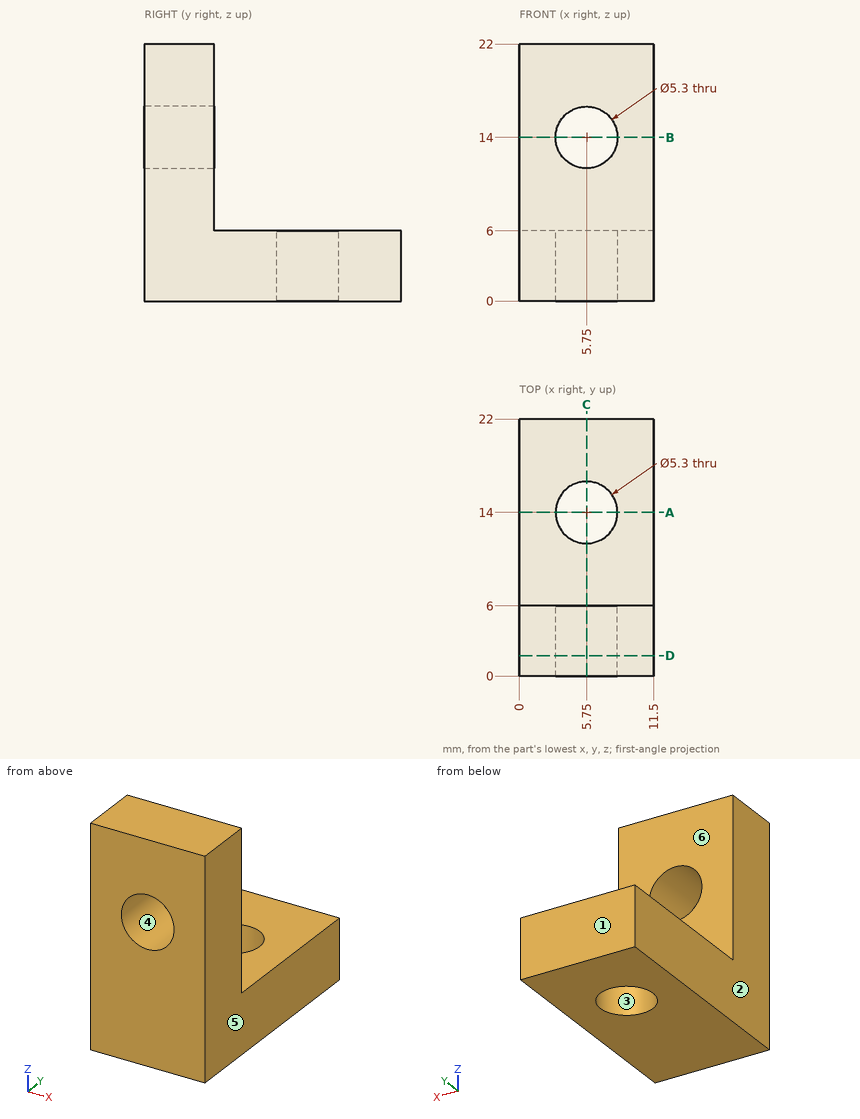
Job drawing, mm, ordinate dimensions from the low corner. One solid piece. A direction names the side the tool comes from. Give positions to 0.01 mm unless a question says otherwise; leave off trailing zeros. Order: outer loops, then holes, each group sorted by start corner. A loop starts at its lowest first (then second) coordinate and runs counter-clockwise, first axis right, second up. Notation, with made-up numbers: M 56,-2.5 L 85,-2.5 A24 ccw 85,28.5 Z; hole C 88.25,-2 d1. An arc over 180 degrees is marked long. Put each result on its own line as item: value. Start each with the question number.
(1) Tool access for the marked faces 5 and 6: list every direction of +Z, -Z, +X, -X, +Y, -Y with a clear straight run to the whole face (end or side of a thin tool).
(2) Band-saw the part on D-D on y = 1.75. Give the cut face in (x, z), then the cut area to 3 significant figures.
(3) Drill centre lines: L1, parallel to X at y = 4.25, z = 14; L2, parallel to Y at x = 10.25, z = 13. Where is each one in solid material? Low to high. Write a range as [from, to].
(4) Pin check, flat tips, straight feed: pin 1 Ø3 at (x, z) = (5.75, 14) entering from +Y; pin 2 Ø4 at (x, z) = (1.5, 17) entering from +Y. Stop position of each tip, or through.
(5) Band-saw the part on A-A on y = 14. Give the cut face in (x, z), then the cut area to 3 significant figures.
(6) Band-saw the part on C-C on x = 5.75. Give the cut face in (y, z), then the cut area to 3 significant figures.
(7) Pull direction X, two halves, no side cores. Call the marked faces 1, 2, 3 and 4: released by +X, released by -X, zero draft, split by the parting line, or undercut.
Results below:
1. face 5: +Z, -Z, +X, +Y, -Y
1. face 6: +Z, +X, -X, +Y
2. outline: M 0,0 L 11.5,0 L 11.5,22 L 0,22 Z; hole C 5.75,14 d5.3
2. area: 231 mm2
3. L1: x = [0, 3.1], [8.4, 11.5]
3. L2: y = [0, 6]
4. pin 1: passes through
4. pin 2: stops at y = 6
5. outline: M 0,0 L 3.1,0 L 3.1,6 L 0,6 Z; M 8.4,0 L 11.5,0 L 11.5,6 L 8.4,6 Z
5. area: 37.2 mm2
6. outline: M 0,0 L 11.35,0 L 11.35,6 L 6,6 L 6,11.35 L 0,11.35 Z; M 0,16.65 L 6,16.65 L 6,22 L 0,22 Z; M 16.65,0 L 22,0 L 22,6 L 16.65,6 Z
6. area: 164 mm2
7. face 1: zero draft
7. face 2: released by -X
7. face 3: undercut
7. face 4: undercut
